Verification items for the finished model (mm, model axes). A direction names the side the tool comes from. Give positions to 0.01 mm unless a question says otherwise; leave off trailing zeros. Order: outer loops, then holes, each group sorted by start corner. A loop starts at its lowest first (then second) coordinate and runs counter-clockwise, first axis right, second up.
(1) Gauge pin test, flat ends, axial feed: pin 1 (5 mm diameter, centred on x = 5.5, z = 8.5, fed in from +Y); pin 2 (2.5 mm diameter, centred on x = 0, y = 8.001, fed in from -Z); pin 3 (0.8 mm diameter, centred on y = 0.5, z = 2, fed in from -X); pin 4 (1.4 mm diameter, centred on y = 8, z = 3, fed in from +X). Record the tip position at first contact, or that the pin passes through.
(2) Sectioned sample at B-B on y = 0. Record the cut outline in (x, z).
(3) Access from +Z, -Z, +X, -X, +Y, -Y to the whole of each face (thin tool, end or side, straight path). Record for faces 1 (the face through (5, 14.605, 3)), 2 (the face through (0.21, 17.62, 3.21)), 3 (the face through (-5, 14.605, 3)), 4 (the face through (4.79, 10.28, 9.37)).
(4) Sectioned sample at C-C on z = 2.75. Count the separate pieces of the cut face and the enclosed holes in it, plus the area to 3 significant figures.
(5) Sectioned sample at D-D on z = 8. Record the cut outline in (x, y).
(6) Sectioned sample at A-A on x = 0. Record the cut outline in (y, z).
(7) Mould release check, pull along X, two halves, no side actions. Record for faces 5 (the face through (3.472, 22.482, 9.37)), 6 (the face through (-8.001, -4, 3)), 7 (the face through (5, -1.397, 3)): pulls with the +X half, pulls with the -X half, needs draft (parallel to the pull), parting line crosses it, or undercut.
(8) Scan lines: L1, parallel to Y at x = -5.75, z = 2.25 (3 decimals); L2, parallel to Y at x = 3, z = 8; L3, parallel to X at y = 0, z = 3.75. Record each from-to range of solid material in increasing order.
```python
from build123d import *

# Parameters (mm, degrees)
SKETCH1_W                 = 16.002
SKETCH1_H                 = 13.208
BOSS_EXTRUDE1_DEPTH       = 6.5024
SKETCH2_W                 = 5.6134
SKETCH2_H                 = 2.794
CUT_EXTRUDE1_DEPTH        = 13.243774857
F_4_CLEARANCE_HOLE1_D     = 3.2639
SKETCH5_R                 = 2.54
BOSS_EXTRUDE2_DEPTH       = 5.8166
SKETCH6_W                 = 16.002
SKETCH6_H                 = 5.207
CUT_EXTRUDE2_DEPTH        = 13.243774857
LPATTERN1_COUNT           = 4
LPATTERN1_PITCH           = 8.001
LPATTERN1_COPY_1_SKETCH_W = 5.6134
LPATTERN1_COPY_1_SKETCH_H = 2.794
LPATTERN1_COPY_1_DEPTH    = 13.243774857
LPATTERN1_COPY_2_SKETCH_W = 5.6134
LPATTERN1_COPY_2_SKETCH_H = 2.794
LPATTERN1_COPY_2_DEPTH    = 13.243774857
LPATTERN1_COPY_3_SKETCH_W = 5.6134
LPATTERN1_COPY_3_SKETCH_H = 2.794
LPATTERN1_COPY_3_DEPTH    = 13.243774857
LPATTERN1_COPY_4_SKETCH_R = 2.54
LPATTERN1_COPY_4_DEPTH    = 5.8166
LPATTERN1_COPY_5_SKETCH_R = 2.54
LPATTERN1_COPY_5_DEPTH    = 5.8166
LPATTERN1_COPY_6_SKETCH_R = 2.54
LPATTERN1_COPY_6_DEPTH    = 5.8166
SKETCH7_W                 = 16.002
SKETCH7_H                 = 8.001
CUT_EXTRUDE3_DEPTH        = 33.296836622


with BuildPart() as part:
    # Sketch1 → Boss-Extrude1 (new body)
    with BuildSketch(Plane.XY):
        Rectangle(SKETCH1_W, SKETCH1_H)
    boss_extrude1 = extrude(amount=BOSS_EXTRUDE1_DEPTH)

    # Sketch2 → Cut-Extrude1 (cut, through all)
    with BuildSketch(Plane.XY.offset(6.5024)):
        with Locations((5.1943, 0)):
            Rectangle(SKETCH2_W, SKETCH2_H)
    cut_extrude1 = extrude(amount=-CUT_EXTRUDE1_DEPTH, mode=Mode.SUBTRACT)

    # #4 Clearance Hole1 (through all)
    with Locations(Plane.XY.offset(6.5024)):
        with Locations((0, 0)):
            f_4_clearance_hole1 = Hole(F_4_CLEARANCE_HOLE1_D / 2)

    # Sketch5 → Boss-Extrude2 (add)
    with BuildSketch(Plane.XY.offset(6.5024)):
        with Locations(Location((2.921, -4.0005, 0), (0, 0, 180))):
            Circle(SKETCH5_R)
    boss_extrude2 = extrude(amount=BOSS_EXTRUDE2_DEPTH)

    # Sketch6 → Cut-Extrude2 (cut, through all)
    with BuildSketch(Plane.XY.offset(6.5024)):
        with Locations((0, 4.0005)):
            Rectangle(SKETCH6_W, SKETCH6_H)
    extrude(amount=-CUT_EXTRUDE2_DEPTH, mode=Mode.SUBTRACT)

    # Mirror4: Cut-Extrude1, Boss-Extrude2 across plane
    add(cut_extrude1.mirror(Plane(origin=(0, 0, 0), x_dir=(0, 0, 1), z_dir=(1, 0, 0))), mode=Mode.SUBTRACT)
    add(boss_extrude2.mirror(Plane(origin=(0, 0, 0), x_dir=(0, 0, 1), z_dir=(1, 0, 0))))

    # LPattern1: Boss-Extrude1, Cut-Extrude1, #4 Clearance Hole1, Boss-Extrude2 ×4
    with Locations(*[(0, i * LPATTERN1_PITCH, 0) for i in range(1, LPATTERN1_COUNT)]):
        add(boss_extrude1)
        add(cut_extrude1, mode=Mode.SUBTRACT)
        add(f_4_clearance_hole1, mode=Mode.SUBTRACT)
        add(boss_extrude2)

    # LPattern1 copy 1 sketch → LPattern1 copy 1 (cut, through all)
    with BuildSketch(Plane(origin=(0, 8.001, 6.5024), x_dir=(-1, 0, 0), z_dir=(0, 0, 1))):
        with Locations((5.1943, 0)):
            Rectangle(LPATTERN1_COPY_1_SKETCH_W, LPATTERN1_COPY_1_SKETCH_H)
    extrude(amount=-LPATTERN1_COPY_1_DEPTH, mode=Mode.SUBTRACT)

    # LPattern1 copy 2 sketch → LPattern1 copy 2 (cut, through all)
    with BuildSketch(Plane(origin=(0, 16.002, 6.5024), x_dir=(-1, 0, 0), z_dir=(0, 0, 1))):
        with Locations((5.1943, 0)):
            Rectangle(LPATTERN1_COPY_2_SKETCH_W, LPATTERN1_COPY_2_SKETCH_H)
    extrude(amount=-LPATTERN1_COPY_2_DEPTH, mode=Mode.SUBTRACT)

    # LPattern1 copy 3 sketch → LPattern1 copy 3 (cut, through all)
    with BuildSketch(Plane(origin=(0, 24.003, 6.5024), x_dir=(-1, 0, 0), z_dir=(0, 0, 1))):
        with Locations((5.1943, 0)):
            Rectangle(LPATTERN1_COPY_3_SKETCH_W, LPATTERN1_COPY_3_SKETCH_H)
    extrude(amount=-LPATTERN1_COPY_3_DEPTH, mode=Mode.SUBTRACT)

    # LPattern1 copy 4 sketch → LPattern1 copy 4 (add)
    with BuildSketch(Plane(origin=(0, 8.001, 6.5024), x_dir=(-1, 0, 0), z_dir=(0, 0, 1))):
        with Locations((2.921, 4.0005)):
            Circle(LPATTERN1_COPY_4_SKETCH_R)
    extrude(amount=LPATTERN1_COPY_4_DEPTH)

    # LPattern1 copy 5 sketch → LPattern1 copy 5 (add)
    with BuildSketch(Plane(origin=(0, 16.002, 6.5024), x_dir=(-1, 0, 0), z_dir=(0, 0, 1))):
        with Locations((2.921, 4.0005)):
            Circle(LPATTERN1_COPY_5_SKETCH_R)
    extrude(amount=LPATTERN1_COPY_5_DEPTH)

    # LPattern1 copy 6 sketch → LPattern1 copy 6 (add)
    with BuildSketch(Plane(origin=(0, 24.003, 6.5024), x_dir=(-1, 0, 0), z_dir=(0, 0, 1))):
        with Locations((2.921, 4.0005)):
            Circle(LPATTERN1_COPY_6_SKETCH_R)
    extrude(amount=LPATTERN1_COPY_6_DEPTH)

    # Sketch7 → Cut-Extrude3 (cut, through all)
    with BuildSketch(Plane.XY.offset(6.5024)):
        with Locations((0, 26.6065)):
            Rectangle(SKETCH7_W, SKETCH7_H)
    extrude(amount=-CUT_EXTRUDE3_DEPTH, mode=Mode.SUBTRACT)


solid = part.part
```
Ans:
1. pin 1: stops at y = 22.61
1. pin 2: passes through
1. pin 3: stops at x = -2.39
1. pin 4: stops at x = 2.39
2. outline: (-2.39, 0) - (-1.63, 0) - (-1.63, 6.5) - (-2.39, 6.5) - close; (1.63, 0) - (2.39, 0) - (2.39, 6.5) - (1.63, 6.5) - close
3. face 1: +Z, -Z, +X
3. face 2: +Z, -Z
3. face 3: +Z, -Z, -X
3. face 4: +Z
4. separate pieces: 1
4. enclosed holes: 3
4. area: 348 mm2
5. outline: circle Ø5.08 at (-2.92, -4); circle Ø5.08 at (-2.92, 4); circle Ø5.08 at (-2.92, 12); circle Ø5.08 at (-2.92, 20); circle Ø5.08 at (2.92, -4); circle Ø5.08 at (2.92, 4); circle Ø5.08 at (2.92, 12); circle Ø5.08 at (2.92, 20)
6. outline: (-6.6, 0) - (-1.63, 0) - (-1.63, 6.5) - (-6.6, 6.5) - close; (1.4, 0) - (6.37, 0) - (6.37, 6.5) - (1.4, 6.5) - close; (9.63, 0) - (14.37, 0) - (14.37, 6.5) - (9.63, 6.5) - close; (17.63, 0) - (22.37, 0) - (22.37, 6.5) - (17.63, 6.5) - close
7. face 5: undercut
7. face 6: pulls with the -X half
7. face 7: needs draft
8. L1: y = -6.604 to -1.397, 1.397 to 6.604, 9.398 to 14.605, 17.399 to 22.606
8. L2: y = -6.54 to -1.46, 1.46 to 6.54, 9.46 to 14.54, 17.46 to 22.54
8. L3: x = -2.39 to -1.63, 1.63 to 2.39
